Verification items for the finished model (mm, model axes). Face numbers are marked on the shaded views. Give positions to 0.01 mm unless a question says otherwise; leave off trailing zeros. Order: outer loops, then holes, each group sorted by start corner. A loop starts at its lowest first (then second) coordinate and runs counter-clockwise, first axis right, second up. Notation, with made-up numbers: M 25.25,66 L 78.25,66 A14 ccw 78.25,71 Z; hole C 59.5,69 d7. An arc over 180 degrees is marked long. Answer as a JSON object with one key per item and string values.
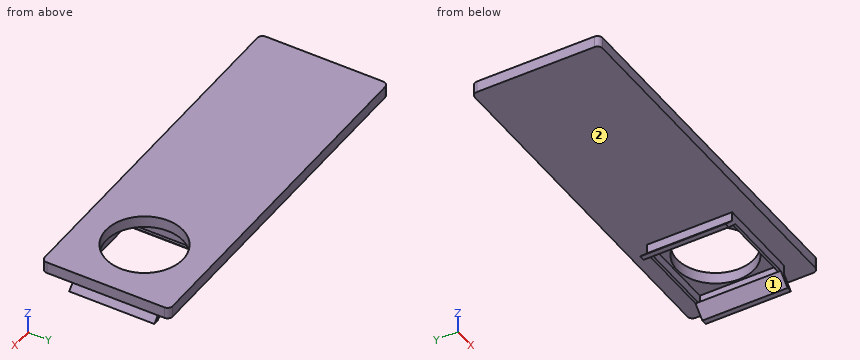
Autodesk Inventor part; units mm, degrees
ref_plane "YZ Plane" through (0, 0, 0) normal (1, 0, 0) x (0, 1, 0)
ref_plane "XZ Plane" through (0, 0, 0) normal (0, 1, 0) x (-1, 0, 0)
ref_plane "XY Plane" through (0, 0, 0) normal (0, 0, 1) x (1, 0, 0)
sketch "Sketch1" plane through (0, 0, 0) normal (0, 0, 1) x (1, 0, 0)
  circle A0 centre (44.9, 4.9) radius 1.45 construction
  circle A1 centre (4.9, 4.9) radius 1.45 construction
  line L0 (2, 2) -> (2, 41.8) construction
  line L1 (47.8, 2) -> (2, 2) construction
  line L2 (47.8, 41.8) -> (47.8, 2) construction
  line L3 (41.8, 41.8) -> (47.8, 41.8) construction
  line L4 (41.8, 8) -> (41.8, 41.8) construction
  line L5 (8, 8) -> (41.8, 8) construction
  line L6 (8, 8) -> (8, 41.8) construction
  line L7 (2, 41.8) -> (8, 41.8) construction
  circle A2 centre (44.9, 44.9) radius 1.4 construction
  circle A3 centre (4.9, 44.9) radius 1.4 construction
  line L8 (2, 47.8) -> (47.8, 47.8) construction
  line L9 (2, 41.8) -> (2, 47.8) construction
  line L10 (47.8, 41.8) -> (2, 41.8) construction
  line L11 (47.8, 41.8) -> (47.8, 47.8) construction
  circle A4 centre (25.6838, 25.4066) radius 13.6 construction
  line L12 (44.1319, 49.8) -> (5.6681, 49.8) construction
  arc A5 (49.8, 47.8) -> (47.8, 49.8) centre (47.8, 47.8) ccw construction
  line L13 (49.8, 41.8) -> (49.8, 47.8) construction
  arc A6 (2, 49.8) -> (0, 47.8) centre (2, 47.8) ccw construction
  arc A7 (0, 2) -> (2, 0) centre (2, 2) ccw construction
  arc A8 (47.8, 0) -> (49.8, 2) centre (47.8, 2) ccw construction
  line L14 (49.8, 0) -> (-90.2, 0)
  line L15 (-90.2, 0) -> (-90.2, 49.8)
  line L16 (-90.2, 49.8) -> (49.8, 49.8)
  line L17 (49.8, 49.8) -> (49.8, 0)
  line L18 (8, 3.7577) -> (41.8, 3.7577) construction
  line L19 (41.8, 0) -> (41.8, 3.7577) construction
  line L20 (8, 0) -> (41.8, 0) construction
  line L21 (8, 0) -> (8, 3.7577) construction
  line L22 (46.1838, 8) -> (46.1838, 41.8) construction
  line L23 (49.8, 41.8) -> (46.1838, 41.8) construction
  line L24 (49.8, 8) -> (49.8, 41.8) construction
  line L25 (46.1838, 8) -> (49.8, 8) construction
  line L26 (3.6162, 41.8) -> (3.6162, 8) construction
  line L27 (0, 8) -> (3.6162, 8) construction
  line L28 (0, 8) -> (0, 41.8) construction
  line L29 (3.6162, 41.8) -> (0, 41.8) construction
  circle A9 centre (24.9, 24.9) radius 15
  arc A10 (42.3945, 24.4616) -> (22.4616, 42.2293) centre (24.9, 24.9) ccw construction
  arc A11 (22.5619, 16.1033) -> (42.3945, 24.4616) centre (29.0002, 28.5351) ccw construction
  line L30 (22.5619, 16.1033) -> (22.3031, 15.1374) construction
  arc A12 (22.3031, 15.1374) -> (41.5232, 19.4302) centre (29.3361, 28.8218) ccw construction
  arc A13 (15.3425, 10.2404) -> (41.5232, 19.4302) centre (24.9, 24.9) ccw construction
  arc A14 (18.2047, 31.6263) -> (15.3425, 10.2404) centre (25.6173, 19.7498) ccw construction
  line L31 (18.2047, 31.6263) -> (17.4976, 32.3335) construction
  arc A15 (17.4976, 32.3335) -> (11.1478, 14.0775) centre (25.6302, 19.2725) ccw construction
  arc A16 (16.2809, 40.1303) -> (11.1478, 14.0775) centre (24.9, 24.9) ccw construction
  arc A17 (34.0602, 27.4798) -> (16.2809, 40.1303) centre (20.0844, 26.6568) ccw construction
  line L32 (34.0602, 27.4798) -> (35.0261, 27.7386) construction
  arc A18 (35.0261, 27.7386) -> (22.4616, 42.2293) centre (19.6533, 27.1018) ccw construction
  line L33 (3.6577, 41.7) -> (8.1, 46.1423) construction
  line L34 (0, 41.7) -> (3.6577, 41.7) construction
  line L35 (0, 8.1) -> (0, 41.7) construction
  line L36 (3.6577, 8.1) -> (0, 8.1) construction
  line L37 (8.1, 3.6577) -> (3.6577, 8.1) construction
  line L38 (8.1, 0) -> (8.1, 3.6577) construction
  line L39 (41.7, 0) -> (8.1, 0) construction
  line L40 (41.7, 3.6577) -> (41.7, 0) construction
  line L41 (46.1423, 8.1) -> (41.7, 3.6577) construction
  line L42 (49.8, 8.1) -> (46.1423, 8.1) construction
  line L43 (49.8, 41.7) -> (49.8, 8.1) construction
  line L44 (46.1423, 41.7) -> (49.8, 41.7) construction
  line L45 (41.7, 46.1423) -> (46.1423, 41.7) construction
  line L46 (41.7, 49.8) -> (41.7, 46.1423) construction
  line L47 (8.1, 49.8) -> (41.7, 49.8) construction
  line L48 (8.1, 46.1423) -> (8.1, 49.8) construction
  circle A19 centre (24.9, 24.9) radius 16.9 construction
  point P0 (0, 0)
  dimension "d0" = 30
  dimension "d4" = 140
extrude "Extrusion1" add sketch "Sketch1" along normal blind 4.5
fillet "Fillet1" radius 2 4 edges at (49.8, 49.8, 2.25) (-90.2, 49.8, 2.25) (49.8, 0, 2.25) (-90.2, 0, 2.25)
sketch "Sketch2" plane through (0, 0, 0) normal (0, 0, -1) x (-1, 0, 0)
  line L0 (-41.8, 8) -> (-41.8, 41.8) construction
  line L1 (-8, 8) -> (-41.8, 8) construction
  line L2 (-8, 8) -> (-8, 41.8) construction
  line L3 (-47.8, 41.8) -> (-2, 41.8) construction
  circle A0 centre (-24.9, 24.9) radius 15 construction
  arc A1 (88.2, 0) -> (90.2, 2) centre (88.2, 2) ccw construction
  line L4 (90.2, 2) -> (90.2, 47.8) construction
  arc A2 (90.2, 47.8) -> (88.2, 49.8) centre (88.2, 47.8) ccw construction
  line L5 (88.2, 49.8) -> (-47.8, 49.8) construction
  arc A3 (-47.8, 49.8) -> (-49.8, 47.8) centre (-47.8, 47.8) ccw construction
  line L6 (-49.8, 47.8) -> (-49.8, 2) construction
  arc A4 (-49.8, 2) -> (-47.8, 0) centre (-47.8, 2) ccw construction
  line L7 (-47.8, 0) -> (88.2, 0) construction
  line L8 (-41.5, 41.5) -> (-8.3, 41.5)
  line L9 (-8.3, 41.5) -> (-8.3, 8.3)
  line L10 (-8.3, 8.3) -> (-41.5, 8.3)
  line L11 (-41.5, 8.3) -> (-41.5, 41.5)
  line L12 (-9.3, 40.5) -> (-40.5, 40.5)
  line L13 (-40.5, 40.5) -> (-40.5, 9.3)
  line L14 (-40.5, 9.3) -> (-9.3, 9.3)
  line L15 (-9.3, 9.3) -> (-9.3, 40.5)
  point P0 (0, 0)
  dimension "d6" = 0.3
  dimension "d7" = 0.3
  dimension "d8" = 0.3
  dimension "d9" = 0.3
  dimension "d10" = 1
extrude "Extrusion2" add sketch "Sketch2" along normal blind 3.66
sketch "Sketch3" plane through (8.3, 8.3, 0) normal (0, -1, 0) x (1, 0, 0)
  line L0 (0, 0) -> (33.2, 0) construction
  line L1 (0, 0) -> (0, -3.66) construction
  line L2 (33.2, -3.66) -> (0, -3.66) construction
  line L3 (33.2, 0) -> (33.2, -3.66) construction
  line L4 (33.5, -3.7577) -> (33.5, -8) construction
  line L5 (-0.3, -8) -> (33.5, -8) construction
  line L6 (-0.3, -3.7577) -> (-0.3, -8) construction
  line L7 (33.5, -3.7577) -> (-0.3, -3.7577) construction
  line L8 (33.5, 0) -> (33.5, -3.6162) construction
  line L9 (-0.3, -3.6162) -> (-0.3, 0) construction
  line L10 (33.2, 0) -> (33.2, -3.66) construction
  line L11 (33.2, 0) -> (33.2, -3.66) construction
  line L12 (33.5, -8) -> (33.5, -3.7577) construction
  line L13 (33.5, -3.7577) -> (-0.3, -3.7577) construction
  line L14 (-0.3, -3.7577) -> (-0.3, -8) construction
  line L15 (-0.3, -8) -> (-4.6838, -8) construction
  line L16 (-2.886, -6.2022) -> (-4.6838, -8) construction
  arc A0 (-2.886, -6.2022) -> (-2.0978, -5.414) centre (-3.4, -4.9) ccw construction
  line L17 (-0.3, -3.6162) -> (-2.0978, -5.414) construction
  line L18 (-0.3, -3.6162) -> (-0.3, 0) construction
  line L19 (-0.3, 0) -> (33.5, 0) construction
  line L20 (33.5, 0) -> (33.5, -3.6162) construction
  line L21 (35.2978, -5.414) -> (33.5, -3.6162) construction
  arc A1 (35.2978, -5.414) -> (36.086, -6.2022) centre (36.6, -4.9) ccw construction
  line L22 (37.8838, -8) -> (36.086, -6.2022) construction
  line L23 (37.8838, -8) -> (33.5, -8) construction
  line L24 (0, -3.66) -> (33.2, -3.66)
  line L25 (0, -3.66) -> (-4.34, -8)
  line L26 (-4.34, -8) -> (-2.2187, -8)
  line L27 (-2.2187, -8) -> (2.1213, -3.66)
  line L28 (16.6, -3.7577) -> (16.6, -8) construction
  line L29 (2.1213, -3.66) -> (0, -3.66)
  line L30 (1, -3.66) -> (32.2, -3.66)
  line L31 (33.5, -3.7577) -> (33.5, -8) construction
  line L32 (33.5, -3.7577) -> (33.5, -8) construction
  line L33 (33.5, -8) -> (37.8838, -8) construction
  line L34 (36.086, -6.2022) -> (37.8838, -8) construction
  arc A2 (35.2978, -5.414) -> (36.086, -6.2022) centre (36.6, -4.9) ccw construction
  line L35 (33.5, -3.6162) -> (35.2978, -5.414) construction
  line L36 (33.2, -3.66) -> (37.54, -8)
  line L37 (37.54, -8) -> (35.4187, -8)
  line L38 (35.4187, -8) -> (31.0787, -3.66)
  line L39 (31.0787, -3.66) -> (33.2, -3.66)
  point P0 (-8.3, 0)
  point P1 (32.2, -3.66)
  dimension "d13" = 1.5
extrude "Extrusion3" add sketch "Sketch3" against normal up to surface (33.2 mm away)
equation "\"d7\" = d6"
equation "\"d8\" = d6"
equation "\"d9\" = d6"
properties part number "30_Smartphone_Holder_v3"
Q1. Material ranges on L1, parallel to X at y = 13, z = -0.75; L2, parallel to Y at x = 24.9, z = 1.95; L3, parallel to Z at x = -65, y = 40.5, recorded low to high.
Resolved:
{"L1": "x = 8.3 to 9.3, 40.5 to 41.5", "L2": "y = 0 to 9.9, 39.9 to 49.8", "L3": "z = 0 to 4.5"}
Q2. Section check D-D on x = -26.5. Record the cut outline in (y, z), then the cut area to 3 significant figures.
Resolved:
{"outline": "M 0,0 L 49.8,0 L 49.8,4.5 L 0,4.5 Z", "area": "224 mm²"}
Q3. Section check C-C on y = 45.5. Record the cut outline in (x, z).
Resolved:
{"outline": "M -90.2,0 L 49.8,0 L 49.8,4.5 L -90.2,4.5 Z"}
Q4. Gauge pin test, flat ends, axial feed: pin 1 Ø12 at (x, y) = (17, 32.5) entering from -Z; pin 2 Ø1.1 at (y, z) = (27, -1.5) entering from -X; pin 3 Ø2 at (y, z) = (39.5, -3) entering from -X; pin 4 Ø4 at (y, z) = (5.5, -3) entering from -X. Record the tip position at first contact, or that the pin passes through.
Resolved:
{"pin 1": "stops at z = 0", "pin 2": "stops at x = 8.3", "pin 3": "stops at x = 7.96", "pin 4": "passes through"}
Q5. Section check B-B on y = 24.9. Record the cut outline in (x, z), then the cut area to 3 significant figures.
Resolved:
{"outline": "M -90.2,0 L 8.3,0 L 8.3,-3.66 L 3.96,-8 L 6.08,-8 L 10.42,-3.66 L 9.3,-3.66 L 9.3,0 L 9.9,0 L 9.9,4.5 L -90.2,4.5 Z; M 39.38,-3.66 L 43.72,-8 L 45.84,-8 L 41.5,-3.66 L 41.5,0 L 49.8,0 L 49.8,4.5 L 39.9,4.5 L 39.9,0 L 40.5,0 L 40.5,-3.66 Z", "area": "521 mm²"}
Q6. Release check for a two-part mould opening along X. For the marked faces 1 and 2 record: +X half, -X half, draft (parallel to the pull), parting line (faces both ways), or undercut.
Resolved:
{"face 1": "undercut", "face 2": "draft"}
Q7. Section check A-A on x = 24.9. Record the cut outline in (y, z), then the cut area to 3 significant figures.
Resolved:
{"outline": "M 0,0 L 8.3,0 L 8.3,-3.66 L 9.3,-3.66 L 9.3,0 L 9.9,0 L 9.9,4.5 L 0,4.5 Z; M 39.9,0 L 40.5,0 L 40.5,-3.66 L 41.5,-3.66 L 41.5,0 L 49.8,0 L 49.8,4.5 L 39.9,4.5 Z", "area": "96.4 mm²"}
